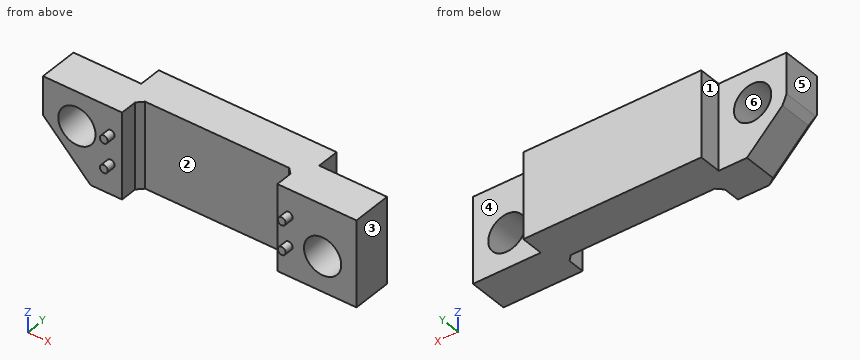
Autodesk Inventor part; units mm, degrees
ref_plane "YZ Plane" through (0, 0, 0) normal (1, 0, 0) x (0, 1, 0)
ref_plane "XZ Plane" through (0, 0, 0) normal (0, 1, 0) x (-1, 0, 0)
ref_plane "XY Plane" through (0, 0, 0) normal (0, 0, 1) x (1, 0, 0)
sketch "Sketch1" plane through (0, 0, 0) normal (0, 1, 0) x (-1, 0, 0)
  line L0 (0, 0) -> (17.75, 0)
  line L1 (17.75, 0) -> (17.75, -7)
  line L2 (17.75, -7) -> (0, -7)
  line L3 (0, -7) -> (0, 0)
  dimension "d0" = 17.75
  dimension "d1" = 7
extrude "Extrusion1" add sketch "Sketch1" along normal blind 2
sketch "Sketch2" plane through (0, 0, 0) normal (0, -1, 0) x (1, 0, 0)
  line L0 (-17.75, 0) -> (0, 0)
  line L1 (0, -7) -> (-17.75, -7)
  line L2 (0, 0) -> (-2, 0)
  line L3 (-2, 0) -> (-2, -7)
  line L4 (-2, -7) -> (0, -7)
  line L5 (0, -7) -> (0, 0)
  line L6 (-17.75, -7) -> (-17.75, 0)
  line L7 (-17.75, 0) -> (-15.75, 0)
  line L8 (-15.75, 0) -> (-15.75, -7)
  line L9 (-15.75, -7) -> (-17.75, -7)
  line L10 (-17.75, -7) -> (-17.75, 0)
  dimension "d4" = 2
  dimension "d5" = 2
extrude "Extrusion2" add sketch "Sketch2" along normal blind 2 contours L0 L8 L1 L6 | L0 L5 L1 L3
sketch "Sketch3" plane through (0, -2, 0) normal (0, -1, 0) x (1, 0, 0)
  line L0 (0, 0) -> (-1, 0)
  line L1 (0, 0) -> (-2, 0)
  line L2 (-1, 0) -> (-1, -2.334)
  line L3 (-1, 0) -> (-1, -4.915)
  circle A0 centre (-1, -2.334) radius 0.35
  circle A1 centre (-1, -4.915) radius 0.35
  line L4 (0, 0) -> (0, -7)
  line L5 (-17.75, -7) -> (-17.75, 0)
  line L6 (0, 0) -> (-17.75, 0)
  line L7 (-15.75, 0) -> (-2, 0)
  line L8 (-8.875, 0) -> (-8.875, -0.7455)
  circle A2 centre (-16.75, -2.334) radius 0.35
  circle A3 centre (-16.75, -4.915) radius 0.35
  dimension "d8" = 1
  dimension "d9" = 2.334
  dimension "d10" = 4.915
  dimension "d11" = 0.7
  dimension "d12" = 0.7
extrude "Extrusion3" add sketch "Sketch3" along normal blind 0.8
sketch "Sketch4" plane through (0, 2, -7) normal (0, 0, -1) x (-1, 0, 0)
  line L0 (0, 0) -> (0, -4)
  line L1 (0, -4) -> (-4, -4)
  line L2 (-4, -4) -> (-4, -2)
  line L3 (-4, -2) -> (0, -2)
  line L4 (0, -2) -> (0, -4)
  line L5 (17.75, -4) -> (17.75, 0)
  line L6 (17.75, -4) -> (21.75, -4)
  line L7 (21.75, -4) -> (21.75, -2)
  line L8 (21.75, -2) -> (17.75, -2)
  line L9 (17.75, -2) -> (17.75, -4)
  dimension "d19" = 4
  dimension "d20" = 2
  dimension "d21" = 4
  dimension "d22" = 2
extrude "Extrusion4" add sketch "Sketch4" against normal blind 7
sketch "Sketch6" plane through (0, 0, -7) normal (0, 1, 0) x (1, 0, 0)
  line L0 (0, -7) -> (0, 0)
  line L1 (4, 0) -> (4, -7)
  line L2 (0, -7) -> (4, -7)
  line L3 (4, -7) -> (4, 0)
  line L4 (4, 0) -> (0, 0)
  line L5 (0, 0) -> (0, -7)
  line L6 (-15.75, -7) -> (-21.75, -7)
  line L7 (0, 0) -> (-17.75, 0)
  line L8 (-21.75, -7) -> (-17.75, -7)
  line L9 (-17.75, -7) -> (-17.75, 0)
  line L10 (-17.75, 0) -> (-21.75, 0)
  line L11 (-21.75, 0) -> (-21.75, -7)
extrude "Extrusion5" add sketch "Sketch6" along normal blind 2
sketch "Sketch8" plane through (0, 2, 0) normal (0, 1, 0) x (1, 0, 0)
  line L0 (4, 0) -> (4, 7)
  line L1 (4, 0) -> (5, 0)
  line L2 (5, 0) -> (5, 7)
  line L3 (5, 7) -> (4, 7)
  line L4 (4, 7) -> (4, 0)
  line L5 (-21.75, 7) -> (-21.75, 0)
  line L6 (-21.75, 0) -> (-22.75, 0)
  line L7 (-22.75, 0) -> (-22.75, 7)
  line L8 (-22.75, 7) -> (-21.75, 7)
  line L9 (-21.75, 7) -> (-21.75, 0)
  point P0 (0, 0)
  dimension "d33" = 1
  dimension "d34" = 1
extrude "Extrusion6" add sketch "Sketch8" against normal blind 4
sketch "Sketch9" plane through (0, 2, 0) normal (0, 1, 0) x (1, 0, 0)
  line L0 (-2, 0) -> (5, 0)
  line L1 (5, 0) -> (2, 0)
  line L2 (2, 0) -> (2, 4.5)
  line L3 (2, 4.5) -> (5, 4.5)
  line L4 (5, 4.5) -> (5, 0)
  line L5 (-22.75, 0) -> (5, 0)
  line L6 (-22.75, 0) -> (-19.75, 0)
  line L7 (-19.75, 0) -> (-19.75, 3)
  line L8 (-19.75, 3) -> (-22.75, 3)
  line L9 (-22.75, 3) -> (-22.75, 0)
  circle A0 centre (2, 4.5) radius 1.65
  circle A1 centre (-19.75, 3) radius 1.65
  point P0 (0, 0)
  dimension "d37" = 3
  dimension "d38" = 4.5
  dimension "d39" = 3
  dimension "d40" = 3
  dimension "d41" = 3.3
  dimension "d42" = 3.3
extrude "Extrusion7" cut sketch "Sketch9" against normal blind 4 contours A0 L3 L2 | L2 L3 A0 | A1 L8 L7 | L7 L8 A1
sketch "Sketch10" plane through (0, 2, 0) normal (0, 1, 0) x (1, 0, 0)
  line L0 (9.5944, -4.5178) -> (-29.7564, -4.5178)
  line L1 (-29.7564, -4.5178) -> (-29.7564, 11.1864)
  line L2 (-29.7564, 11.1864) -> (9.5944, 11.1864)
  line L3 (9.5944, 11.1864) -> (9.5944, -4.5178)
  point P0 (0, 0)
extrude "Extrusion8" cut sketch "Sketch10" against normal blind 0.5
sketch "Sketch11" plane through (0, 1.5, 0) normal (0, 1, 0) x (1, 0, 0)
  circle A0 centre (2, 4.5) radius 1.65
  line L0 (2, 4.5) -> (-1, 4.5)
  circle A1 centre (-19.75, 3) radius 1.65
  line L1 (-19.75, 3) -> (-16.75, 3)
  line L2 (-16.75, 3) -> (-16.75, 7.7148)
  line L3 (-22.75, 7) -> (5, 7)
  line L4 (5, 0) -> (-22.75, 0)
  line L5 (-16.75, 7) -> (-1, 7)
  line L6 (-1, 7) -> (-1, 0)
  line L7 (-1, 0) -> (-16.75, 0)
  line L8 (-16.75, 0) -> (-16.75, 7)
  point P0 (0, 0)
  point P1 (-16.75, 0)
  point P2 (-1, 7)
  dimension "d47" = 3
  dimension "d48" = 3
extrude "Extrusion9" add sketch "Sketch11" along normal blind 2 contours L2 L3 L6 L4 L8
chamfer "Chamfer1" distance 0.5 angle 45 2 edges at (-2, 0, -3.5) (-15.75, 0, -3.5)
sketch "Sketch12" plane through (0, -2, 0) normal (0, -1, 0) x (1, 0, 0)
  line L0 (-15.75, 0) -> (-15.75, -7)
  line L1 (-15.75, -7) -> (-22.75, -7)
  line L2 (-15.75, 0) -> (-17.75, 0)
  line L3 (-17.75, 0) -> (-17.75, -7)
  line L4 (-17.75, -7) -> (-15.75, -7)
  line L5 (-15.75, -7) -> (-15.75, 0)
  line L6 (-22.75, 0) -> (-22.75, -7)
  line L7 (-17.75, -7) -> (-22.75, -7)
  line L8 (-22.75, -7) -> (-22.75, 0)
  line L9 (-22.75, 0) -> (-17.75, 0)
  line L10 (-17.75, 0) -> (-17.75, -7)
  point P0 (0, 0)
  dimension "d57" = 2
sketch "Sketch13" plane through (-15.75, -2, -7) normal (0, 0, -1) x (-1, 0, 0)
  line L0 (0, 0) -> (7, 0)
  line L1 (1, 3.5) -> (7, 3.5)
  line L2 (0, 0) -> (7, 0)
  line L3 (7, 0) -> (7, 3.5)
  line L4 (7, 3.5) -> (0, 3.5)
  line L5 (0, 1.5) -> (0, 0)
  line L6 (-13.75, 0) -> (-20.75, 0)
  line L7 (-20.75, 3.5) -> (-20.75, 0)
  line L8 (-13.75, 0) -> (-20.75, 0)
  line L9 (-20.75, 0) -> (-20.75, 3.5)
  line L10 (-20.75, 3.5) -> (-13.75, 3.5)
  line L11 (-14.75, 5.5) -> (1, 5.5)
  line L12 (-14.75, 5.5) -> (1, 5.5)
  line L13 (1, 5.5) -> (1, 2)
  line L14 (-14.75, 2) -> (-14.75, 5.5)
  line L15 (0, 1.5) -> (-0.5, 2)
  line L16 (0, 1.5) -> (-0.5, 2)
  line L17 (-13.75, 1.5) -> (-13.75, 0)
  line L18 (-13.25, 2) -> (-13.75, 1.5)
  line L19 (-13.75, 1.5) -> (-13.25, 2)
  line L20 (-13.75, 1.5) -> (-13.75, 0)
  line L21 (-0.5, 2) -> (-13.25, 2)
  point P0 (-15.75, 2)
  point P1 (-14.75, 3.5)
extrude "Extrusion10" add sketch "Sketch13" along normal blind 0.6
chamfer "Chamfer3" distance 3.5 angle 45 1 edges at (-22.75, -0.25, -7.6)
chamfer "Chamfer4" distance 0.5 angle 45 1 edges at (-21, -2, -5.85)
chamfer "Chamfer5" distance 0.5 angle 45 1 edges at (-22.75, 0, -4.1)
properties part number "IMU_clamp"
CAD build for the part. Positions are in the model's coordinates, mm. Face numbers are marked on the shaded views. A direction names the side the tool comes from. Round coordinates to 2 decimals unless told otherwise and drop trailing zeros. Loops run counter-clockwise (first coordinate to the right, second up) from the corner with the lowest first, then second, coordinate; pieces in that order, holes last.
(1) Cut at C-C (x = -7.25). Give the cut face in (y, z), plus the area to 3 significant figures.
(2) Drop flat-ended pins along their axis: pin 1 (3 mm diameter, centred on x = 2.5, z = -3, fed in from +Y); pin 2 (1.6 mm diameter, centred on y = 2.5, z = -3, fed in from +X); pin 3 (0.6 mm diameter, centred on y = 2.5, z = -2, fed in from -X). Give the stop position or say it passes through.
(3) Wall check: line 1 along Z through (x, y) = (2, 0.1); line 2 along Z through (x, y) = (-16.75, -2.5) (3 decimals); line 3 along X through (y, z) = (0.55, -4.5). Give the ranges that are in metal, low to high.
(4) Which spindle directions (+Z, -Z, +X, -X, +Y, -Y) get a long thin tool onto all of the face, cutting with end or side? Do the marked faces 1, 2 and 3. Say none if no direction does.
(5) Cut at B-B (x = 2). Give the cut face in (y, z), plus the area to 4 significant figures.
(6) Cut at D-D (y = 3). Give the cut face in (x, z), plus the area to 3 significant figures.
(7) Two-plate mould, pull along X, no slides. Class the marked faces 4, 5 and 6: +X half, -X half, draft (parallel to the pull), parting line (faces both ways), or undercut.
(8) Cut at A-A (y = -0.25). Give the cut face in (x, z).
Findings below:
1. outline: (0, -7.6) - (3.5, -7.6) - (3.5, 0) - (0, 0) - close
1. area: 26.6 mm2
2. pin 1: stops at y = 1.5
2. pin 2: stops at x = -1
2. pin 3: stops at x = -16.75
3. line 1: z = -7.6 to -6.15, -2.85 to 0
3. line 2: z = -5.265 to -4.565, -2.684 to -1.984
3. line 3: x = -22.35 to -20.44, -19.06 to 0.35, 3.65 to 5
4. face 1: +Z, -Z, -X, +Y
4. face 2: +Z, -Z, -Y
4. face 3: +Z, -Z, +X, +Y, -Y
5. outline: (-2, -7.6) - (1.5, -7.6) - (1.5, -6.15) - (-2, -6.15) - close; (-2, -2.85) - (1.5, -2.85) - (1.5, 0) - (-2, 0) - close
5. area: 15.05 mm2
6. outline: (-16.75, -7.6) - (-1, -7.6) - (-1, 0) - (-16.75, 0) - close
6. area: 120 mm2
7. face 4: draft
7. face 5: -X half
7. face 6: undercut
8. outline: (-22.75, -3.6) - (-22.4, -4.45) - (-19.25, -7.6) - (-15.5, -7.6) - (-15.5, 0) - (-22.75, 0) - close; (-2.25, -7.6) - (5, -7.6) - (5, 0) - (-2.25, 0) - close; hole circle Ø3.3 at (-19.75, -3); hole circle Ø3.3 at (2, -4.5)
